Read the model definition and answer for the solid it produces. Units are mm, in the model's axes. Coordinates: 2 decimals unless noted, no trailing zeros. Loops run counter-clockwise (first coordinate to the right, second up) from the corner with the lowest first, then second, coordinate; pieces in that order, holes last.
from build123d import *

# Parameters (mm, degrees)
SKETCH1_R           = 1.016
SKETCH1_R_2         = 1.5875
SKETCH1_W           = 4.7625
SKETCH1_H           = 3.175
BOSS_EXTRUDE2_DEPTH = 3.175


with BuildPart() as part:
    # Sketch1 → Boss-Extrude2 (new body)
    with BuildSketch(Plane(origin=(0, 0, 0), x_dir=(1, 0, 0), z_dir=(0, 1, 0))):
        with BuildLine():
            Line((-18.264134833, 18.784590512), (-73.66, 18.784590512))
            ThreePointArc((-73.66, 18.784590512), (-75.456051224, 18.040641736), (-76.2, 16.244590512))
            Line((-76.2, 16.244590512), (-76.2, 9.196090512))
            Line((-76.2, 9.196090512), (-73.025, 9.196090512))
            Line((-73.025, 9.196090512), (-73.025, 6.021090512))
            Line((-73.025, 6.021090512), (-76.2, 6.021090512))
            Line((-76.2, 6.021090512), (-76.2, -43.994090512))
            Line((-76.2, -43.994090512), (-48.493603884, -59.990385768))
            ThreePointArc((-48.493603884, -59.990385768), (-46.566203509, -60.244132842), (-45.023899358, -59.060681243))
            Line((-45.023899358, -59.060681243), (-22.163899358, -19.465999782))
            ThreePointArc((-22.163899358, -19.465999782), (-20.621595207, -18.282548183), (-18.694194832, -18.536295256))
            Line((-18.694194832, -18.536295256), (-7.155626979, -25.198090512))
            Line((-7.155626979, -25.198090512), (20.55218651, -73.189431243))
            ThreePointArc((20.55218651, -73.189431243), (22.094490662, -74.372882842), (24.021891036, -74.119135768))
            Line((24.021891036, -74.119135768), (30.126071095, -70.594885768))
            Line((30.126071095, -70.594885768), (28.538571095, -67.845255111))
            Line((28.538571095, -67.845255111), (31.288201752, -66.257755111))
            Line((31.288201752, -66.257755111), (32.875701752, -69.007385768))
            Line((32.875701752, -69.007385768), (76.2, -43.994090512))
            Line((76.2, -43.994090512), (76.2, -12.0015))
            ThreePointArc((76.2, -12.0015), (75.456051224, -10.205448776), (73.66, -9.4615))
            Line((73.66, -9.4615), (27.94, -9.4615))
            ThreePointArc((27.94, -9.4615), (26.143948776, -8.717551224), (25.4, -6.9215))
            Line((25.4, -6.9215), (25.4, 6.4135))
            Line((25.4, 6.4135), (53.097932583, 54.387726499))
            ThreePointArc((53.097932583, 54.387726499), (53.351679656, 56.315126873), (52.168228058, 57.857431024))
            Line((52.168228058, 57.857431024), (46.064047999, 61.381681024))
            Line((46.064047999, 61.381681024), (44.476547999, 58.632050367))
            Line((44.476547999, 58.632050367), (41.726917342, 60.219550367))
            Line((41.726917342, 60.219550367), (43.314417342, 62.969181024))
            Line((43.314417342, 62.969181024), (-0.009880906, 87.982476281))
            Line((-0.009880906, 87.982476281), (-27.706396116, 71.991885768))
            ThreePointArc((-27.706396116, 71.991885768), (-28.889847715, 70.449581617), (-28.636100642, 68.522181243))
            Line((-28.636100642, 68.522181243), (-5.776100642, 28.927499782))
            ThreePointArc((-5.776100642, 28.927499782), (-5.522353569, 27.000099407), (-6.705805168, 25.457795256))
            Line((-6.705805168, 25.457795256), (-18.264134833, 18.784590512))
        make_face()
        with Locations((69.2404, -28.829)):
            Circle(SKETCH1_R, mode=Mode.SUBTRACT)
        with Locations((-59.586846366, -45.549445368)):
            Circle(SKETCH1_R, mode=Mode.SUBTRACT)
        with Locations((-9.653553634, 74.378445368)):
            Circle(SKETCH1_R, mode=Mode.SUBTRACT)
        with Locations((22.2504, -28.829)):
            Circle(SKETCH1_R, mode=Mode.SUBTRACT)
        with Locations((-36.091846366, -4.854911644)):
            Circle(SKETCH1_R, mode=Mode.SUBTRACT)
        with Locations((13.841446366, 33.683911644)):
            Circle(SKETCH1_R, mode=Mode.SUBTRACT)
        with Locations((26.738386423, -61.552243797)):
            Circle(SKETCH1_R_2, mode=Mode.SUBTRACT)
        with Locations((20.388386423, -50.553721169)):
            Circle(SKETCH1_R_2, mode=Mode.SUBTRACT)
        with Locations((-53.975, 7.608590512)):
            Circle(SKETCH1_R_2, mode=Mode.SUBTRACT)
        with Locations((-66.675, 7.608590512)):
            Circle(SKETCH1_R_2, mode=Mode.SUBTRACT)
        with Locations((33.576732671, 42.928016425)):
            Circle(SKETCH1_R_2, mode=Mode.SUBTRACT)
        with Locations((39.926732671, 53.926539053)):
            Circle(SKETCH1_R_2, mode=Mode.SUBTRACT)
        Polygon((14.251071095, -43.098579198), (16.632321095, -47.223025184), (19.381951752, -45.635525184), (17.000701752, -41.511079198), align=None, mode=Mode.SUBTRACT)
        with Locations((-46.83125, 7.62)):
            Rectangle(SKETCH1_W, SKETCH1_H, mode=Mode.SUBTRACT)
        Polygon((29.830548248, 39.603025184), (27.449298248, 35.478579198), (30.198928905, 33.891079198), (32.580178905, 38.015525184), align=None, mode=Mode.SUBTRACT)
    extrude(amount=BOSS_EXTRUDE2_DEPTH)


solid = part.part
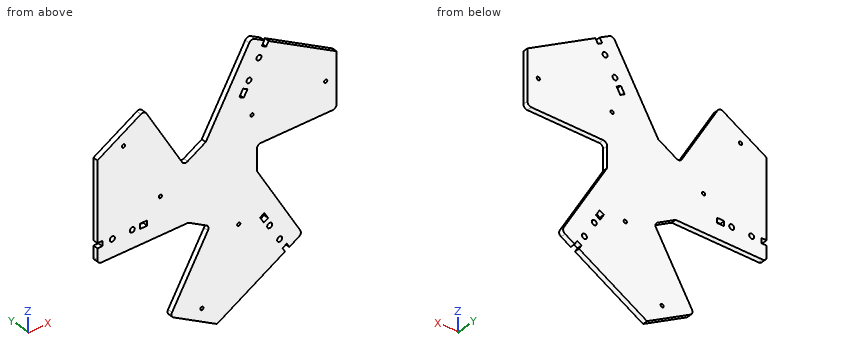
Item 1: A cutting plane is placed at B-B on z = 2. Determine the outline of the cut face in (x, y) (3 decimals).
Numbers:
outline: (-76.2, 0) - (25.4, 0) - (25.4, 3.175) - (-76.2, 3.175) - close
Item 2: A cutting plane is placed at C-C on y = 2.2. Give the number of separate pieces and of enclosed holes in the cut face, then the cut area to 3 significant figures.
Numbers:
separate pieces: 1
enclosed holes: 15
area: 12,500 mm2
Item 3: A cutting plane is placed at A-A on x = 48.5. Determine the outline of the cut face in (y, z) (1 decimal), then the cut area to 3 significant figures.
Numbers:
outline: (0, -60) - (3.2, -60) - (3.2, -46.4) - (0, -46.4) - close; (0, 9.5) - (3.2, 9.5) - (3.2, 60) - (0, 60) - close
area: 203 mm2
Item 4: Given pin 1 (1 mm diameter, centred on x = -48, y = 2, fed in from +Z); pin 2 (3 mm diameter, centred on x = -66.68, z = -7.61, fed in from -Y); pin 3 (1 mm diameter, centred on y = 2, z = -8, fed in from +X); pin 4 (1.6 mm diameter, centred on y = 2, z = -7.5, fed in from -X) (3 decimals), each flat-ended and moving along its own axis, determine where each tip first touches the part or whether it passes through.
Numbers:
pin 1: stops at z = 60.32
pin 2: passes through
pin 3: stops at x = 26.6
pin 4: stops at x = -73.025
Item 5: Find the intervals of material crossed by line 1 along Z through (x, y) = (39, 1.1); line 2 along X through (y, z) = (2.45, 50); line 3 along Z through (x, y) = (42, 1.6), in increasing order.
Numbers:
line 1: z = -65.46 to -55.22, -52.64 to -29.97, 9.46 to 65.47
line 2: x = -65.8 to -39.79, 7.16 to 18.9, 21.88 to 65.8
line 3: z = -63.73 to -60.69, -60.06 to -35.17, 9.46 to 63.74
Item 6: A cutting plane is placed at D-D on x = -31.5. Determine the outline of the cut face in (y, z) (3 decimals), then the cut area to 3 significant figures.
Numbers:
outline: (0, -18.785) - (3.175, -18.785) - (3.175, 35.637) - (0, 35.637) - close
area: 173 mm2
